from build123d import *

# Parameters (mm, degrees)
BOSS_EXTRU_1_DEPTH      = 30
ENL_V_MAT_EXTRU_1_REACH = 247.316
ESQUISSE3_R             = 5.832843768
ESQUISSE3_R_2           = 5.351266955
ENL_V_MAT_EXTRU_2_DEPTH = 236.071663242


with BuildPart() as part:
    # Esquisse1 → Boss.-Extru.1 (new body)
    with BuildSketch(Plane.XY):
        Polygon((-14.050192106, 18.448375062), (-4.050192106, 18.448375062), (2.761752479, -113.222934174), (135.150414635, -146.982486488), (157.659448917, -129.804321414), (157.659448917, -53.333080108), (168.106392916, -53.333080108), (168.106392916, -144.596025192), (147.431500323, -161.551624938), (-14.050192106, -161.551624938), align=None)
    extrude(amount=BOSS_EXTRU_1_DEPTH)

    # Enlèv. mat.-Extru.1: up to this plane
    enl_v_mat_extru_1_end = Plane(origin=(-4.050192106, 18.448375062, 30), z_dir=(-0.9986644529274081, -0.05166537001900487, 0))
    # Esquisse3 → Enlèv. mat.-Extru.1 (cut, up to the surface)
    with BuildSketch(Plane.ZY.offset(14.050192106), mode=Mode.PRIVATE) as enl_v_mat_extru_1_sk1:
        with Locations((15.037241333, -92.337647956)):
            Circle(ESQUISSE3_R)
    enl_v_mat_extru_1_tool1 = split(extrude(enl_v_mat_extru_1_sk1.sketch, amount=-ENL_V_MAT_EXTRU_1_REACH, mode=Mode.PRIVATE), bisect_by=enl_v_mat_extru_1_end, keep=Keep.BOTH, mode=Mode.PRIVATE)
    add(enl_v_mat_extru_1_tool1.solids().sort_by_distance((-14.050192, -92.337648, 15.037241))[0], mode=Mode.SUBTRACT)
    # Esquisse3 → Enlèv. mat.-Extru.1 (cut, up to the surface)
    with BuildSketch(Plane.ZY.offset(14.050192106), mode=Mode.PRIVATE) as enl_v_mat_extru_1_sk2:
        with Locations((15.037241333, -21.264425603)):
            Circle(ESQUISSE3_R_2)
    enl_v_mat_extru_1_tool2 = split(extrude(enl_v_mat_extru_1_sk2.sketch, amount=-ENL_V_MAT_EXTRU_1_REACH, mode=Mode.PRIVATE), bisect_by=enl_v_mat_extru_1_end, keep=Keep.BOTH, mode=Mode.PRIVATE)
    add(enl_v_mat_extru_1_tool2.solids().sort_by_distance((-14.050192, -21.264426, 15.037241))[0], mode=Mode.SUBTRACT)

    # Esquisse5 → Enlèv. mat.-Extru.2 (cut, through all)
    with BuildSketch(Plane.XY.offset(30)):
        Polygon((-7.286706934, -119.304572357), (133.336369925, -155.163928004), (-7.286706934, -155.163928004), align=None)
    extrude(amount=-ENL_V_MAT_EXTRU_2_DEPTH, mode=Mode.SUBTRACT)


solid = part.part
The listing builds one solid part. Answer for the finished solid, in the listing's coordinates (mm). A direction names the side the tool comes from. Coordinates: 2 decimals unless noted, no trailing zeros. Write each loop counter-clockwise with the first axis right and the second up, starting at its lowest first coordinate (ties: lowest second). Pieces come first, ordered by that corner, then holes. Notation, with made-up numbers: (72, 54.5) - (119, 54.5) arc R11 cw to (119, 58.5) - close; hole circle Ø11 at (-38.5, -34.75). An arc over 180 degrees is marked (long way). Put each result on its own line as item: value.
1. The part is cut by section D-D on x = 10.5. Give the vertices of the cut face in (y, z).
Answer sheet:
outline: (-161.55, 0) - (-155.16, 0) - (-155.16, 30) - (-161.55, 30) - close; (-123.84, 0) - (-115.2, 0) - (-115.2, 30) - (-123.84, 30) - close
2. The part is cut by section B-B on y = -150.5. Give the vertices of the cut face in (x, z).
Answer sheet:
outline: (-14.05, 0) - (-7.29, 0) - (-7.29, 30) - (-14.05, 30) - close; (115.05, 0) - (160.91, 0) - (160.91, 30) - (115.05, 30) - close
3. Determine the mould class of faces 4 (the face through (62.04, -136.983, 15.21)), 5 (the face through (68, -161.552, 15)), 6 (the face through (-0.69, -46.47, 14.79)) for opening direction Y: pulls with the +Y half, pulls with the -Y half, needs draft (parallel to the pull), parting line crosses it, or undercut.
Answer sheet:
face 4: undercut
face 5: pulls with the -Y half
face 6: pulls with the +Y half
4. Flat-ended cylindrical pins translate along their axes: pin 1 Ø4 at (x, y) = (83.5, -130) entering from +Z; pin 2 Ø2 at (x, z) = (126.5, 26) entering from +Y; pin 3 Ø12.5 at (y, z) = (-21.26, 15.04) entering from +X; pin 4 Ø3 at (x, z) = (165, 9) entering from +Y. Find the tip coordinate at first contact, or state that the pin passes through.
Answer sheet:
pin 1: passes through
pin 2: stops at y = -144.52
pin 3: stops at x = -1.67
pin 4: stops at y = -53.33
5. The part is cut by section A-A on z = 17.5. Give the vertices of the cut face in (x, y).
Answer sheet:
outline: (-14.05, -161.55) - (147.43, -161.55) - (168.11, -144.6) - (168.11, -53.33) - (157.66, -53.33) - (157.66, -129.8) - (135.15, -146.98) - (2.76, -113.22) - (1.95, -97.63) - (-14.05, -97.63) - close; (-14.05, -87.05) - (1.41, -87.05) - (-1.75, -26.02) - (-14.05, -26.02) - close; (-14.05, -16.51) - (-2.24, -16.51) - (-4.05, 18.45) - (-14.05, 18.45) - close; hole (-7.29, -155.16) - (133.34, -155.16) - (-7.29, -119.3) - close
6. The part is cut by section C-C on z = 6. Give the vertices of the cut face in (x, y).
Answer sheet:
outline: (-14.05, -161.55) - (147.43, -161.55) - (168.11, -144.6) - (168.11, -53.33) - (157.66, -53.33) - (157.66, -129.8) - (135.15, -146.98) - (2.76, -113.22) - (-4.05, 18.45) - (-14.05, 18.45) - close; hole (-7.29, -155.16) - (133.34, -155.16) - (-7.29, -119.3) - close
7. Find the intervals of material crossed by line 1 along Y through (x, z) = (121, 24); line 2 along X through (y, z) = (-53.5, 14); line 3 along Y through (x, z) = (50.5, 22.5), in increasing order. Write a range as from..to.
Answer sheet:
line 1: y = -161.55..-155.16, -152.02..-143.37
line 2: x = -14.05..-0.33, 157.66..168.11
line 3: y = -161.55..-155.16, -134.04..-125.4
8. A tool of negligible diameter and unlimited length cuts with its end or side. For faces 1 (the face through (-6.12, -97.51, 17.73)), 2 (the face through (157.659, -92, 15)), 3 (the face through (-7.287, -137, 15)), from which of +Z, -Z, +X, -X, +Y, -Y can it reach the whole face along a straight path? Write none if from no direction.
Answer sheet:
face 1: -X
face 2: +Z, -Z, +Y
face 3: +Z, -Z
